Model file for the job. Use its own axes, mm. Face numbers are marked on the shaded views. A direction names the side the tool comes from. Give positions to 0.01 mm unless a question says otherwise; leave off trailing zeros. Order: outer loops, then holes, each group sorted by start corner. A loop starts at its lowest first (then second) coordinate and runs counter-clockwise, first axis right, second up. Notation, with made-up numbers: M 5.25,85.25 L 43.25,85.25 A14 cw 43.25,96.25 Z; hole C 52,18.25 d10. An arc over 180 degrees is marked long. Return JSON: item names as keys, results as strings. Group by question number.
1. Two-plate mould, pull along X, no slides. Class the marked faces 4, 5 and 6: released by +X, released by -X, zero draft, split by the parting line, or undercut.
2. 3-axis set-ups, long thin cutter, end or side, ignore diameter. For the marked faces 1, 2 and 3: which of +Z, -Z, +X, -X, +Y, -Y reach the whole face in a straight line?
3. Pin check, flat tips, straight feed: pin 1 (3 mm diameter, centred on x = 0, z = 0, fed in from -Y); pin 2 (1.5 mm diameter, centred on y = 9.5, z = 2, fed in from -X); pin 3 (4 mm diameter, centred on x = 1.5, y = 6.5, fed in from +Z). Stop position of each tip, or through.
4. Wall check: probe 1 along Y at (x, z) = (0, -3.55); probe 2 along Y at (x, z) = (-2, 6.25); probe 3 along X at (y, z) = (2, -2.75). Give the ranges that are in metal, low to high. Write a range as [from, to].
5. Slice it at B-B on x = 0. List the corners of the cut face in (y, z), then the cut area to 3 significant figures.
6. Slice it at A-A on z = 0. List the corners of the cut face in (x, y).
from build123d import *

# Parameters (mm, degrees)
BOSS_EXTRUDE1_DEPTH     = 5.08
BOSS_EXTRUDE1_DRAFT     = -10
SKETCH2_R               = 1.016
CUT_EXTRUDE1_DEPTH      = 6.08
SKETCH3_R               = 1.778
CUT_EXTRUDE2_DEPTH      = 2.032
SKETCH4_R               = 4.3815
CUT_EXTRUDE3_DEPTH      = 2.032
SKETCH3_2_R             = 1.778
CUT_EXTRUDE4_DEPTH      = 10.16
CUT_EXTRUDE4_DEPTH_BACK = 2.032
SKETCH7_R               = 1.5875
CUT_EXTRUDE5_DEPTH      = 11.43
SKETCH8_R               = 0.5
CUT_EXTRUDE6_DEPTH      = 9.181885328


with BuildPart() as part:
    # Sketch1 → Boss-Extrude1 (with draft: the straight prism first)
    with BuildSketch(Plane(origin=(0, 0, 0), x_dir=(1, 0, 0), z_dir=(0, 1, 0))):
        with BuildLine():
            ThreePointArc((7.458830017, -1.558927446), (6.599113577, 3.81), (2.379344237, 7.239))
            ThreePointArc((2.379344237, 7.239), (0, 6.858), (-2.379344237, 7.239))
            ThreePointArc((-2.379344237, 7.239), (-6.599113577, 3.81), (-7.458830017, -1.558927446))
            ThreePointArc((-7.458830017, -1.558927446), (-5.939202219, -3.429), (-5.079485779, -5.680072554))
            ThreePointArc((-5.079485779, -5.680072554), (0, -7.62), (5.079485779, -5.680072554))
            ThreePointArc((5.079485779, -5.680072554), (5.939202219, -3.429), (7.458830017, -1.558927446))
        make_face()
    extrude(amount=BOSS_EXTRUDE1_DEPTH)
    # Boss-Extrude1: the draft: its side faces are tilted about the plane it starts from
    boss_extrude1_sides = [part.faces().sort_by_distance(p)[0] for p in [
        (5.939202219, 2.54, 3.429),
        (6.599113577, 2.54, -3.81),
        (0, 2.54, -6.858),
        (-6.599113577, 2.54, -3.81),
        (-5.939202219, 2.54, 3.429),
        (0, 2.54, 7.62),
    ]]
    draft(boss_extrude1_sides, Plane(origin=(0, 0, 0), x_dir=(1, 0, 0), z_dir=(0, 1, 0)), BOSS_EXTRUDE1_DRAFT)

    # Sketch2 → Cut-Extrude1 (cut, through all)
    with BuildSketch(Plane(origin=(0, 5.08, 0), x_dir=(1, 0, 0), z_dir=(0, 1, 0))):
        with Locations((0, -6.35)):
            Circle(SKETCH2_R)
        with Locations((-5.499261314, 3.175)):
            Circle(SKETCH2_R)
        with Locations((5.499261314, 3.175)):
            Circle(SKETCH2_R)
    extrude(amount=-CUT_EXTRUDE1_DEPTH, mode=Mode.SUBTRACT)

    # Sketch3 → Cut-Extrude2 (cut)
    with BuildSketch(Plane(origin=(0, 5.08, 0), x_dir=(1, 0, 0), z_dir=(0, 1, 0))):
        with Locations((0, -6.35)):
            Circle(SKETCH3_R)
        with Locations((-5.499261314, 3.175)):
            Circle(SKETCH3_R)
        with Locations((5.499261314, 3.175)):
            Circle(SKETCH3_R)
    extrude(amount=-CUT_EXTRUDE2_DEPTH, mode=Mode.SUBTRACT)

    # Sketch4 → Cut-Extrude3 (cut)
    with BuildSketch(Plane.XZ):
        Circle(SKETCH4_R)
    extrude(amount=-CUT_EXTRUDE3_DEPTH, mode=Mode.SUBTRACT)

    # Sketch6 → Revolve1 (revolve)
    with BuildSketch(Plane.XY):
        with BuildLine():
            Line((0, 5.08), (0, 15.24))
            Line((0, 15.24), (4.318, 15.24))
            ThreePointArc((4.318, 15.24), (4.830980871, 10.059396174), (6.35, 5.08))
            Line((6.35, 5.08), (0, 5.08))
        make_face()
    revolve(axis=Axis((0, 5.08, 0), (0, 1, 0)))

    # Sketch3<2> → Cut-Extrude4 (cut, two sides)
    with BuildSketch(Plane(origin=(0, 5.08, 0), x_dir=(1, 0, 0), z_dir=(0, 1, 0))) as cut_extrude4_sk:
        with Locations((0, -6.35)):
            Circle(SKETCH3_2_R)
        with Locations((-5.499261314, 3.175)):
            Circle(SKETCH3_2_R)
        with Locations((5.499261314, 3.175)):
            Circle(SKETCH3_2_R)
    extrude(amount=CUT_EXTRUDE4_DEPTH, mode=Mode.SUBTRACT)
    extrude(cut_extrude4_sk.sketch, amount=-CUT_EXTRUDE4_DEPTH_BACK, mode=Mode.SUBTRACT)

    # Sketch7 → Cut-Extrude5 (cut)
    with BuildSketch(Plane(origin=(0, 15.24, 0), x_dir=(1, 0, 0), z_dir=(0, 1, 0))):
        Circle(SKETCH7_R)
    extrude(amount=-CUT_EXTRUDE5_DEPTH, mode=Mode.SUBTRACT)

    # Sketch8 → Cut-Extrude6 (cut, through all)
    with BuildSketch(Plane.XY):
        with Locations((0, 12.7)):
            Circle(SKETCH8_R)
    extrude(amount=-CUT_EXTRUDE6_DEPTH, mode=Mode.SUBTRACT)


solid = part.part
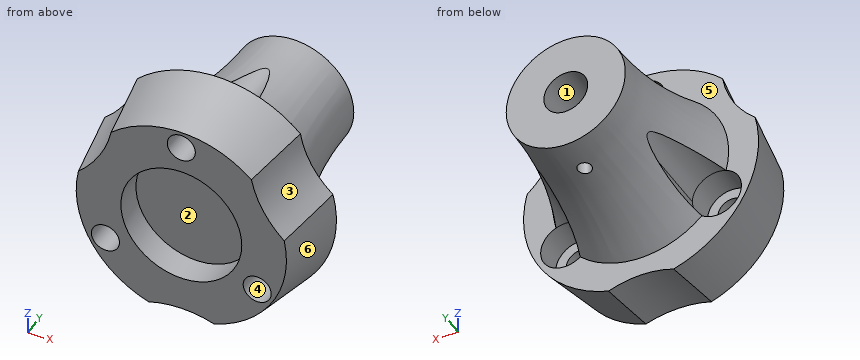
Result:
{
 "1": {"face 4": "undercut", "face 5": "zero draft", "face 6": "released by +X"},
 "2": {"face 1": "+Y", "face 2": "-Y", "face 3": "+Z, +X, -Y"},
 "3": {"pin 1": "stops at y = 2.03", "pin 2": "stops at x = -4.86", "pin 3": "stops at z = 8.52"},
 "4": {"probe 1": "y = [2.03, 12.2], [13.2, 15.24]", "probe 2": "y = [0, 5.08]", "probe 3": "x = [-7.48, -6.42], [-4.58, -3.41], [3.41, 4.58], [6.42, 7.48]"},
 "5": {"outline": "M 0,-6.86 L 5.08,-7.75 L 5.08,-6.35 A26.42 cw 12.2,-4.49 L 12.2,-1.59 L 3.81,-1.59 L 3.81,1.59 L 15.24,1.59 L 15.24,4.32 A26.42 cw 11.59,4.57 L 3.05,4.57 L 3.05,5.33 L 0,5.33 L 0,4.38 L 2.03,4.38 L 2.03,-4.38 L 0,-4.38 Z; M 0,7.37 L 3.05,7.37 L 3.05,8.13 L 5.08,8.13 L 5.08,8.52 L 0,7.62 Z; M 13.2,-4.4 A26.42 cw 15.24,-4.32 L 15.24,-1.59 L 13.2,-1.59 Z", "area": "104 mm2"},
 "6": {"outline": "M -8.52,5.08 L -7.62,0 L -4.38,0 L -4.38,2.03 L 4.38,2.03 L 4.38,0 L 7.62,0 L 8.52,5.08 L 6.35,5.08 A26.42 cw 4.32,15.24 L 1.59,15.24 L 1.59,3.81 L -1.59,3.81 L -1.59,15.24 L -4.32,15.24 A26.42 cw -6.35,5.08 Z"}
}
